Part model, mm, in its own coordinate system. Round coordinates to 2 decimals unless told otherwise and drop trailing zeros. Loops run counter-clockwise (first coordinate to the right, second up) from the corner with the lowest first, then second, coordinate; pieces in that order, holes last.
1) Band-saw the part on D-D, the plane y = 3.65. State how many separate pieces and enclosed holes the cut face has, then the cut area to 3 significant figures.
2) Drop flat-ended pins along their axis: P1, Ø3.5, axis at x = 75.31, z = 17.21, coming from the -Y side; P2, Ø2.5, axis at x = -110.7, z = 3.91, coming from the -Y side; P3, Ø2, axis at y = 4, z = 23, coming from the +X side; P4, Ø1.5, axis at x = 20.5, y = 1.5, coming from the -Z side. Give the stop position or say it passes through.
3) Band-saw the part on B-B, the plane x = -48.5. Write the cut outline in (y, z), then the cut area to 3 significant figures.
4) Band-saw the part on C-C, the plane z = 55. Write the cut outline in (x, y).
5) Band-saw the part on A-A, the plane x = 28. Write the cut outline in (y, z), then the cut area to 3 significant figures.
6) Probe line 1 (Z direction, x = 35.5, y = 2.7); line 2 (Z direction, x = 18, y = 3.25); line 3 (X direction, y = 0.9, z = 11) (3 decimals). List the from-to ranges inside material, lowest first.
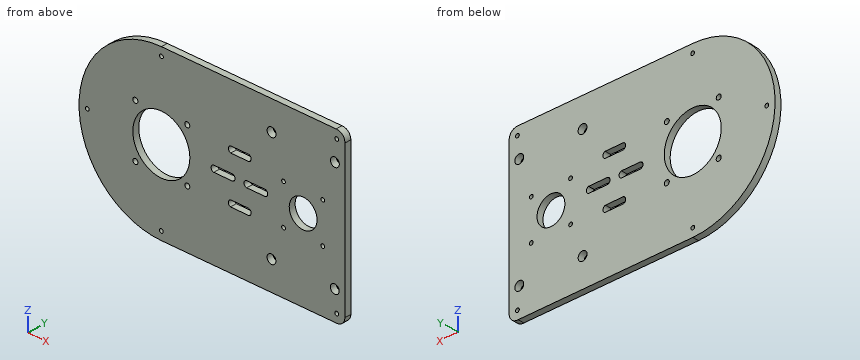
from build123d import *

# Parameters (mm, degrees)
BOSS_EXTRUDE1_DEPTH = 5
SKETCH3_R           = 1.475
CUT_EXTRUDE1_DEPTH  = 137.064643721
SKETCH4_R           = 22.5
SKETCH4_R_2         = 11
SKETCH4_R_3         = 1.975
SKETCH4_R_4         = 1.475
SKETCH4_R_5         = 3.5
CUT_EXTRUDE2_DEPTH  = 137.064643721


with BuildPart() as part:
    # Sketch2 → Boss-Extrude1 (new body)
    with BuildSketch(Plane(origin=(0, 0, 0), x_dir=(1, 0, 0), z_dir=(0, 1, 0))):
        with BuildLine():
            Line((-52.202038886, 61.082677165), (85.797961114, 61.082677165))
            ThreePointArc((85.797961114, 61.082677165), (90.6611457, 59.421487905), (92.797961114, 54.747717054))
            Line((92.797961114, 54.747717054), (92.797961114, -62.252282946))
            ThreePointArc((92.797961114, -62.252282946), (90.782438223, -67.143884297), (85.797961114, -68.917322835))
            Line((85.797961114, -68.917322835), (-52.202038886, -68.917322835))
            ThreePointArc((-52.202038886, -68.917322835), (-117.202038886, -3.917322835), (-52.202038886, 61.082677165))
        make_face()
    extrude(amount=BOSS_EXTRUDE1_DEPTH)

    # Sketch3 → Cut-Extrude1 (cut, through all)
    with BuildSketch(Plane(origin=(0, 5, 0), x_dir=(1, 0, 0), z_dir=(0, 1, 0))):
        with Locations(Location((86.297961114, 54.582677165, 0), (0, 0, 270))):
            Circle(SKETCH3_R)
        with Locations(Location((-52.202038886, 54.582677165, 0), (0, 0, 270))):
            Circle(SKETCH3_R)
        with Locations(Location((-110.702038886, -3.912214457, 0), (0, 0, 270))):
            Circle(SKETCH3_R)
        with Locations(Location((86.297961114, -62.417322835, 0), (0, 0, 90))):
            Circle(SKETCH3_R)
        with Locations(Location((-52.11000774, -62.417322835, 0), (0, 0, 90))):
            Circle(SKETCH3_R)
    extrude(amount=-CUT_EXTRUDE1_DEPTH, mode=Mode.SUBTRACT)

    # Sketch4 → Cut-Extrude2 (cut, through all)
    with BuildSketch(Plane(origin=(0, 5, 0), x_dir=(1, 0, 0), z_dir=(0, 1, 0))):
        with BuildLine():
            Line((17.035736777, 16.673447137), (2.353343762, 16.650369213))
            ThreePointArc((2.353343762, 16.650369213), (0.763165117, 14.196667771), (2.526429623, 11.864240457))
            Line((2.526429623, 11.864240457), (16.842011582, 11.886741824))
            ThreePointArc((16.842011582, 11.886741824), (18.721537255, 14.207947413), (17.035736777, 16.673447137))
        make_face()
        with BuildLine():
            Line((4.221952, -1.260399725), (-10.778048, -1.260399725))
            ThreePointArc((-10.778048, -1.260399725), (-12.893391284, -3.603735064), (-10.910792873, -6.060399725))
            Line((-10.910792873, -6.060399725), (4.221952, -6.060399725))
            ThreePointArc((4.221952, -6.060399725), (6.021952, -3.660399725), (4.221952, -1.260399725))
        make_face()
        with BuildLine():
            Line((30.221952, -1.260399725), (15.221952, -1.260399725))
            ThreePointArc((15.221952, -1.260399725), (13.106608716, -3.603735064), (15.089207127, -6.060399725))
            Line((15.089207127, -6.060399725), (30.147453765, -6.060399725))
            ThreePointArc((30.147453765, -6.060399725), (31.77239266, -3.68504141), (30.221952, -1.260399725))
        make_face()
        with BuildLine():
            Line((16.866686946, -19.510676527), (2.551087303, -19.510676527))
            ThreePointArc((2.551087303, -19.510676527), (0.791491102, -21.845872472), (2.385524529, -24.297071429))
            Line((2.385524529, -24.297071429), (17.06793568, -24.297071429))
            ThreePointArc((17.06793568, -24.297071429), (18.749858786, -21.828924997), (16.866686946, -19.510676527))
        make_face()
        with Locations(Location((-52.181545547, -3.280325568, 0), (0, 0, 270))):
            Circle(SKETCH4_R)
        with Locations(Location((59.810085593, -1.911181789, 0), (0, 0, 270))):
            Circle(SKETCH4_R_2)
        with Locations(Location((-72.707038886, 16.240452632, 0), (0, 0, 270))):
            Circle(SKETCH4_R_3)
        with Locations(Location((-72.707038886, -24.769547368, 0), (0, 0, 270))):
            Circle(SKETCH4_R_3)
        with Locations(Location((-31.697038886, -24.769547368, 0), (0, 0, 90))):
            Circle(SKETCH4_R_3)
        with Locations(Location((-31.697038886, 16.240452632, 0), (0, 0, 90))):
            Circle(SKETCH4_R_3)
        with Locations(Location((44.310085593, 13.788312606, 0), (0, 0, 270))):
            Circle(SKETCH4_R_4)
        with Locations(Location((44.310085593, -17.211687394, 0), (0, 0, 270))):
            Circle(SKETCH4_R_4)
        with Locations(Location((75.310085593, -17.211687394, 0), (0, 0, 90))):
            Circle(SKETCH4_R_4)
        with Locations(Location((75.310085593, 13.788312606, 0), (0, 0, 90))):
            Circle(SKETCH4_R_4)
        with Locations(Location((84.797961114, 38.74145607, 0), (0, 0, 270))):
            Circle(SKETCH4_R_5)
        with Locations(Location((34.797961114, 38.74145607, 0), (0, 0, 270))):
            Circle(SKETCH4_R_5)
        with Locations(Location((84.864762974, -46.25854393, 0), (0, 0, 270))):
            Circle(SKETCH4_R_5)
        with Locations(Location((34.864824738, -46.337134304, 0), (0, 0, 270))):
            Circle(SKETCH4_R_5)
    extrude(amount=-CUT_EXTRUDE2_DEPTH, mode=Mode.SUBTRACT)


solid = part.part
Reported:
1. separate pieces: 1
1. enclosed holes: 23
1. area: 22,900 mm2
2. P1: stops at y = 0
2. P2: passes through
2. P3: stops at x = 92.8
2. P4: stops at z = -61.08
3. outline: (0, -61.08) - (5, -61.08) - (5, -18.92) - (0, -18.92) - close; (0, 25.48) - (5, 25.48) - (5, 68.92) - (0, 68.92) - close
3. area: 428 mm2
4. outline: (-92.4, 0) - (92.8, 0) - (92.8, 5) - (-92.4, 5) - close
5. outline: (0, -61.08) - (5, -61.08) - (5, 1.26) - (0, 1.26) - close; (0, 6.06) - (5, 6.06) - (5, 68.92) - (0, 68.92) - close
5. area: 626 mm2
6. line 1: z = -61.08 to -42.17, -35.31 to 42.9, 49.78 to 68.92
6. line 2: z = -61.08 to -16.07, -12.55 to 1.26, 6.06 to 20.15, 23.72 to 68.92
6. line 3: x = -116.815 to -73.316, -31.047 to 53.614, 66.006 to 92.798
